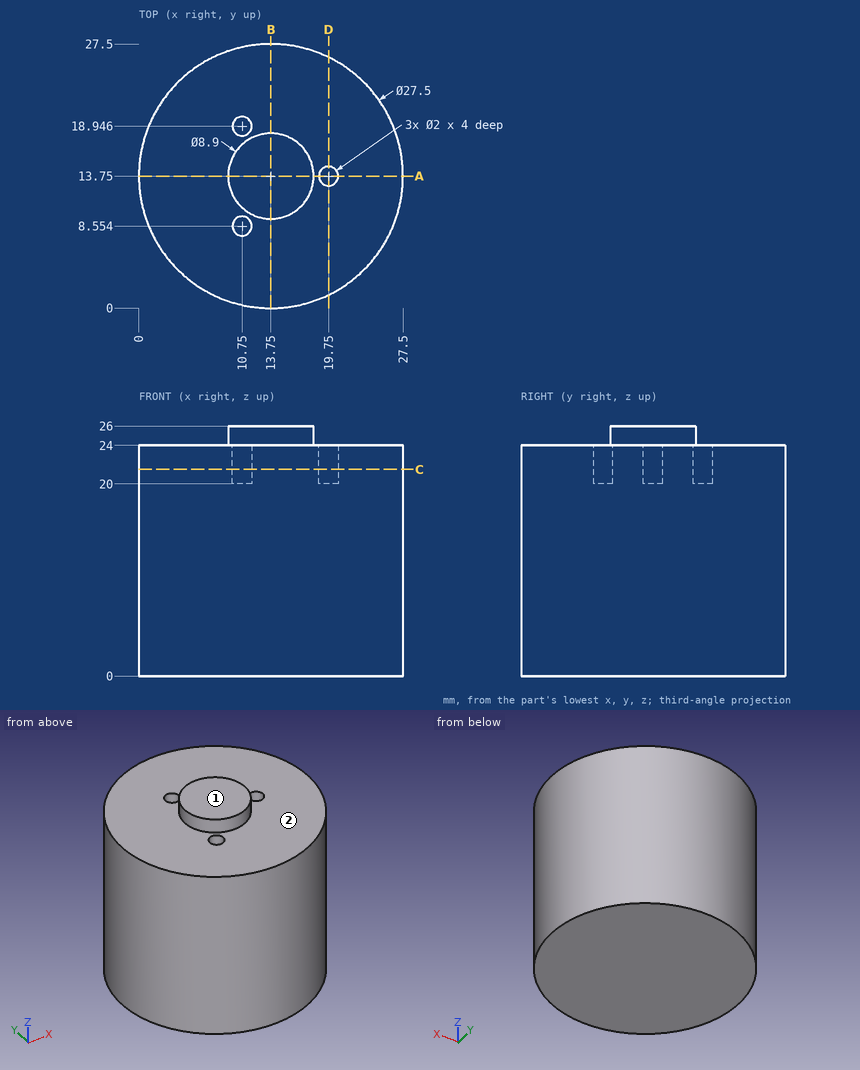
Design review of the part shown in the three views and the two pictorial views. Dimensions are in mm from the part's minimum x, y and z. A direction names the side the tool comes from. Round coordinates to 2 decimals unless told otherwise and drop trailing zeros. Order: outer loops, then holes, each group sorted by start corner. A loop starts at its lowest first (then second) coordinate and runs counter-clockwise, first axis right, second up. Notation, with made-up numbers: (28, 8) -> (68, 8) arc R34 cw to (68, 39) -> close; hole circle Ø4 at (44, -8.5). An arc over 180 degrees is marked (long way). Write item = value, one per line. Start each with the question number.
1) Insertion check: pin 1 (1.6 mm diameter, centred on x = 10.5, y = 8, fed in from +Z); pin 2 (3 mm diameter, centred on x = 6.5, z = 19.5, fed in from -Y); pin 3 (5 mm diameter, centred on x = 21.5, z = 11.5, fed in from -Y). Each pin has a flat end and moves straight along its axis. Give the tip position at first contact, or say it passes through.
2) Take a section at C-C on z = 21.5. State the section outline as (x, y) points.
3) Take a section at B-B on x = 13.75. State the section outline as (y, z) points, plus the area to 3 significant figures.
4) Take a section at A-A on y = 13.75. State the section outline as (x, z) points, plus the area to 3 significant figures.
5) To check wall thickness, follow line 1 (Y direction, x = 10.75, z = 23.2); line 2 (Z direction, x = 4.5, y = 22.25); line 3 (Y direction, x = 19.75, z = 22.9). State the ranges of each line that lie inside material, in increasing order. Write a range as from..to.
6) Tool access review of the marked faces 1 and 2: name each direction out of +Z, -Z, +X, -X, +Y, -Y from which nothing blocks a thin tool from reaching the whole face with its end or side.
7) Take a section at D-D on x = 19.75. State the section outline as (y, z) points, plus the area to 3 significant figures.
Verdict:
q1.pin_1 = 24
q1.pin_2 = 1.26
q1.pin_3 = 1.04
q2.outline = circle Ø27.5 at (13.75, 13.75); hole circle Ø2 at (10.75, 8.55); hole circle Ø2 at (10.75, 18.95); hole circle Ø2 at (19.75, 13.75)
q3.outline = (0, 0) -> (27.5, 0) -> (27.5, 24) -> (18.2, 24) -> (18.2, 26) -> (9.3, 26) -> (9.3, 24) -> (0, 24) -> close
q3.area = 678 mm2
q4.outline = (0, 0) -> (27.5, 0) -> (27.5, 24) -> (20.75, 24) -> (20.75, 20) -> (18.75, 20) -> (18.75, 24) -> (18.2, 24) -> (18.2, 26) -> (9.3, 26) -> (9.3, 24) -> (0, 24) -> close
q4.area = 670 mm2
q5.line_1 = 0.33..7.55, 9.55..17.95, 19.95..27.17
q5.line_2 = 0..24
q5.line_3 = 1.38..12.75, 14.75..26.12
q6.face_1 = +Z, +X, -X, +Y, -Y
q6.face_2 = +Z
q7.outline = (1.38, 0) -> (26.12, 0) -> (26.12, 24) -> (14.75, 24) -> (14.75, 20) -> (12.75, 20) -> (12.75, 24) -> (1.38, 24) -> close
q7.area = 586 mm2
